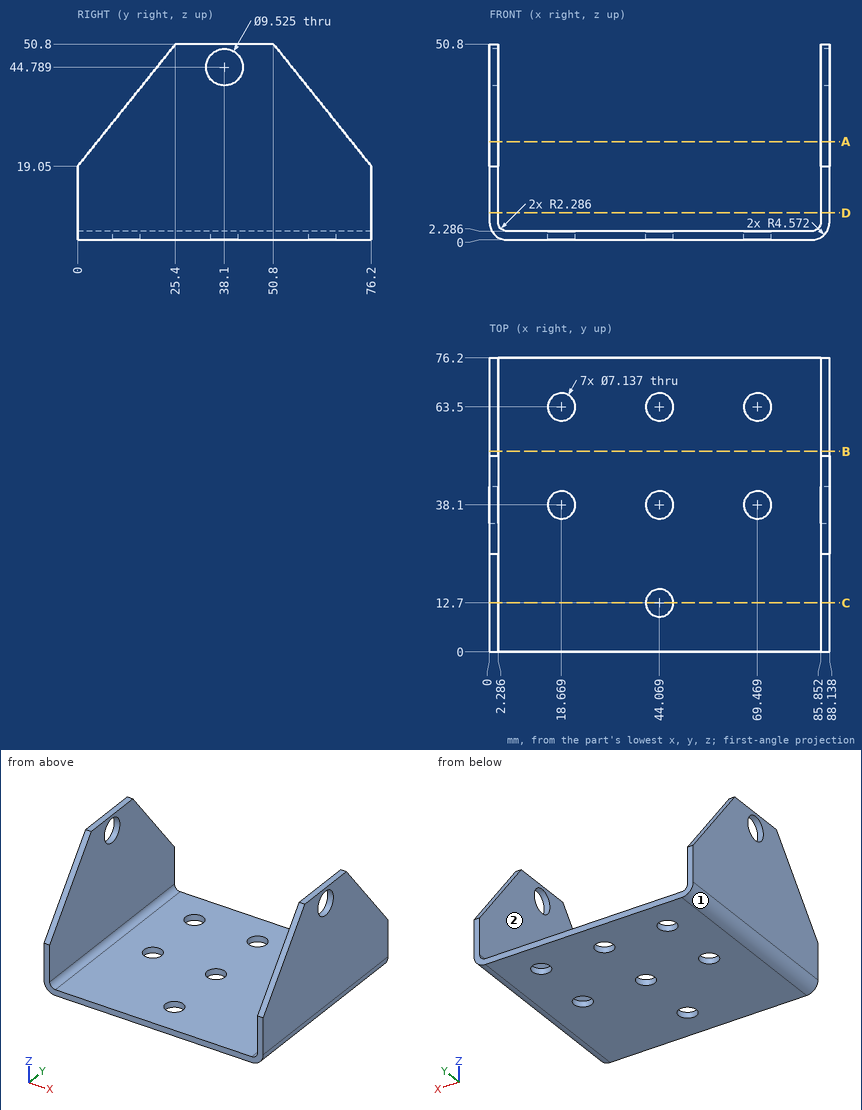
Input: dimensioned drawing with shaded views. Units: mm. Origin: part minimum x, y, z. A direction names the side the tool comes from. Coordinates: 2 decimals unless noted, no trailing zeros. Order: outer loops, then holes, each group sorted by start corner. A loop starts at its lowest first (then second) coordinate and runs counter-clockwise, first axis right, second up.
Item 1: Section query A-A (z = 25.5). Output: boundary loops of the cut face in (x, y), then the cut area to 3 significant figures.
Answer:
outline: (0, 5.16) - (2.29, 5.16) - (2.29, 71.04) - (0, 71.04) - close; (85.85, 5.16) - (88.14, 5.16) - (88.14, 71.04) - (85.85, 71.04) - close
area: 301 mm2
Item 2: Material intervals for line 1 along X through (y, z) = (63, 5.5); line 2 along X through (y, z) = (38, 1) (1 decimal); line 3 along Z through (x, y) = (33.5, 15), sorted ascending.
Answer:
line 1: x = 0 to 2.29, 85.85 to 88.14
line 2: x = 1.7 to 15.1, 22.2 to 40.5, 47.6 to 65.9, 73 to 86.4
line 3: z = 0 to 2.29
Item 3: Contact query for flat-ended pins moving along their axis: P1, Ø11.5, axis at x = 44.069, y = 38.1, coming from the +Z side; P2, Ø8, axis at x = 46, y = 61, coming from the -Z side. Output: stop coordinate, or through.
Answer:
P1: stops at z = 2.29
P2: stops at z = 0
Item 4: Section query B-B (y = 52). Output: boundary loops of the cut face in (x, z).
Answer:
outline: (0, 4.57) arc R4.57 ccw to (4.57, 0) - (83.57, 0) arc R4.57 ccw to (88.14, 4.57) - (88.14, 49.3) - (85.85, 49.3) - (85.85, 4.57) arc R2.29 cw to (83.57, 2.29) - (4.57, 2.29) arc R2.29 cw to (2.29, 4.57) - (2.29, 49.3) - (0, 49.3) - close
Item 5: Section query C-C (y = 12.7). Output: boundary loops of the cut face in (x, z) (1 decimal).
Answer:
outline: (0, 4.6) arc R4.6 ccw to (4.6, 0) - (40.5, 0) - (40.5, 2.3) - (4.6, 2.3) arc R2.3 cw to (2.3, 4.6) - (2.3, 34.9) - (0, 34.9) - close; (47.6, 0) - (83.6, 0) arc R4.6 ccw to (88.1, 4.6) - (88.1, 34.9) - (85.9, 34.9) - (85.9, 4.6) arc R2.3 cw to (83.6, 2.3) - (47.6, 2.3) - close
Item 6: Access query for the marked faces 1 and 2. Directions: +Z, -Z, +X, -X, +Y, -Y. A direction counts if a zero-diameter tool reaches every point of the face in a straight line with its end or side. Return the directions, or none.
Answer:
face 1: -Z, -X, +Y, -Y
face 2: +Z, +Y, -Y
Item 7: Section query D-D (z = 7). Output: boundary loops of the cut face in (x, y).
Answer:
outline: (0, 0) - (2.29, 0) - (2.29, 76.2) - (0, 76.2) - close; (85.85, 0) - (88.14, 0) - (88.14, 76.2) - (85.85, 76.2) - close
